from build123d import *

# Parameters (mm, degrees)
BOSS_EXTRUDE1_DEPTH      = 11
CUT_EXTRUDE1_DEPTH       = 62.923844357
CUT_EXTRUDE1_DEPTH_BACK  = 62.923844357
SKETCH2_W                = 20.5
SKETCH2_H                = 2.6
BOSS_EXTRUDE3_START      = -8.4
BOSS_EXTRUDE3_DEPTH      = 9.4
SKETCH4_R                = 17
SKETCH4_R_2              = 10
BOSS_EXTRUDE2_DEPTH      = 5.62
SKETCH5_R                = 13.5
CUT_EXTRUDE2_DEPTH       = 4
CUT_EXTRUDE3_DEPTH       = 37.67089309
CUT_EXTRUDE3_DEPTH_BACK  = 37.67089309
SKETCH6_R                = 10.5
BOSS_EXTRUDE4_START      = 1.12
SKETCH18_R               = 17
BOSS_EXTRUDE4_DEPTH      = 1.12
CHAMFER3_SIZE            = 2.75
BOSS_EXTRUDE7_START      = 1
BOSS_EXTRUDE7_DEPTH      = 1
CUT_EXTRUDE17_START      = 12
SKETCH28_W               = 22
SKETCH28_H               = 42
CUT_EXTRUDE17_DEPTH      = 11
CUT_EXTRUDE18_DEPTH      = 37.488140539
CUT_EXTRUDE18_DEPTH_BACK = 37.488140539
SKETCH29_R               = 11
SKETCH31_R               = 1.9
CUT_EXTRUDE19_DEPTH      = 7
BOSS_EXTRUDE8_DEPTH      = 3


with BuildPart() as part:
    # Sketch1 → Boss-Extrude1 (new body)
    with BuildSketch(Plane.XY):
        with BuildLine():
            ThreePointArc((15.25, 27.5), (14.664213562, 28.914213562), (13.25, 29.5))
            Line((13.25, 29.5), (-10.25, 29.5))
            ThreePointArc((-10.25, 29.5), (-11.664213562, 28.914213562), (-12.25, 27.5))
            Line((-12.25, 27.5), (-12.25, 0.346410162))
            Line((-12.25, 0.346410162), (-12.25, 0))
            Line((-12.25, 0), (-12.25, -0.346410162))
            Line((-12.25, -0.346410162), (-12.25, -27.5))
            ThreePointArc((-12.25, -27.5), (-11.664213562, -28.914213562), (-10.25, -29.5))
            Line((-10.25, -29.5), (13.25, -29.5))
            ThreePointArc((13.25, -29.5), (14.664213562, -28.914213562), (15.25, -27.5))
            Line((15.25, -27.5), (15.25, -9.120855223))
            Line((15.25, -9.120855223), (15.25, 9.120855223))
            Line((15.25, 9.120855223), (15.25, 27.5))
        make_face()
        with BuildLine():
            Line((7, 22.5), (10.25, 22.5))
            Line((10.25, 22.5), (10.25, -22.5))
            Line((10.25, -22.5), (7, -22.5))
            Line((7, -22.5), (7, -24.7))
            ThreePointArc((7, -24.7), (5, -26.7), (3, -24.7))
            Line((3, -24.7), (3, -22.5))
            Line((3, -22.5), (-3, -22.5))
            Line((-3, -22.5), (-3, -24.7))
            ThreePointArc((-3, -24.7), (-5, -26.7), (-7, -24.7))
            Line((-7, -24.7), (-7, -22.5))
            Line((-7, -22.5), (-10.25, -22.5))
            Line((-10.25, -22.5), (-10.25, 22.5))
            Line((-10.25, 22.5), (-7, 22.5))
            Line((-7, 22.5), (-7, 24.7))
            ThreePointArc((-7, 24.7), (-5, 26.7), (-3, 24.7))
            Line((-3, 24.7), (-3, 22.5))
            Line((-3, 22.5), (3, 22.5))
            Line((3, 22.5), (3, 24.7))
            ThreePointArc((3, 24.7), (5, 26.7), (7, 24.7))
            Line((7, 24.7), (7, 22.5))
        make_face(mode=Mode.SUBTRACT)
    extrude(amount=BOSS_EXTRUDE1_DEPTH)

    # Sketch2 → Cut-Extrude1 (cut, two sides: drawn at the far end of the back side and taken through both)
    with BuildSketch(Plane(origin=(0, 29.5, 0), x_dir=(1, 0, 0), z_dir=(0, 1, 0)).offset(-CUT_EXTRUDE1_DEPTH_BACK)):
        with Locations((0, -1.3)):
            Rectangle(SKETCH2_W, SKETCH2_H)
    extrude(amount=CUT_EXTRUDE1_DEPTH + CUT_EXTRUDE1_DEPTH_BACK, mode=Mode.SUBTRACT)

    # Sketch3 → Boss-Extrude3 (add)
    with BuildSketch(Plane.XY.offset(11).offset(BOSS_EXTRUDE3_START)):
        with BuildLine():
            Line((-10.25, -29.5), (13.25, -29.5))
            ThreePointArc((13.25, -29.5), (14.664213562, -28.914213562), (15.25, -27.5))
            Line((15.25, -27.5), (15.25, 27.5))
            ThreePointArc((15.25, 27.5), (14.664213562, 28.914213562), (13.25, 29.5))
            Line((13.25, 29.5), (-10.25, 29.5))
            ThreePointArc((-10.25, 29.5), (-11.664213562, 28.914213562), (-12.25, 27.5))
            Line((-12.25, 27.5), (-12.25, -27.5))
            ThreePointArc((-12.25, -27.5), (-11.664213562, -28.914213562), (-10.25, -29.5))
        make_face()
    extrude(amount=BOSS_EXTRUDE3_DEPTH)

    # Sketch4 → Boss-Extrude2 (add)
    with BuildSketch(Plane.XY.offset(17.62)):
        with Locations((0, -11.7)):
            Circle(SKETCH4_R)
        with Locations((0, -11.7)):
            Circle(SKETCH4_R_2, mode=Mode.SUBTRACT)
    extrude(amount=-BOSS_EXTRUDE2_DEPTH)

    # Sketch5 → Cut-Extrude2 (cut)
    with BuildSketch(Plane.XY.offset(17.62)):
        with Locations((0, -11.7)):
            Circle(SKETCH5_R)
    extrude(amount=-CUT_EXTRUDE2_DEPTH, mode=Mode.SUBTRACT)

    # Sketch6 → Cut-Extrude3 (cut, two sides: drawn at the far end of the back side and taken through both)
    with BuildSketch(Plane.XY.offset(13.62).offset(-CUT_EXTRUDE3_DEPTH_BACK)):
        with Locations((0, -11.7)):
            Circle(SKETCH6_R)
    extrude(amount=CUT_EXTRUDE3_DEPTH + CUT_EXTRUDE3_DEPTH_BACK, mode=Mode.SUBTRACT)

    # Sketch18 → Boss-Extrude4 (add)
    with BuildSketch(Plane.XY.offset(12).offset(BOSS_EXTRUDE4_START)):
        with Locations((0, -11.7)):
            Circle(SKETCH18_R)
    extrude(amount=-BOSS_EXTRUDE4_DEPTH)

    # Chamfer3
    # the kernel refuses this chamfer: 2.75 mm, written as the material it adds along each edge
    with BuildSketch(Plane(origin=(0, -11.7, 12), x_dir=(0.99914018616096, 0.041459478991448445, 0), z_dir=(0.041459478991448445, -0.99914018616096, 0))) as chamfer3_piece_1_section:
        Polygon((17, CHAMFER3_SIZE), (17 + CHAMFER3_SIZE, 0), (17, 0), align=None)
    chamfer3_piece_1 = revolve(axis=Axis((0, -11.7, 12), (0, 0, 1)), revolution_arc=157.576683104, mode=Mode.PRIVATE)
    chamfer3_piece_1 = split(chamfer3_piece_1, bisect_by=Plane(origin=(15.25, 6.422467161, 13.340102963), z_dir=(-1, 0, 0)), keep=Keep.TOP, mode=Mode.PRIVATE)
    chamfer3_piece_1 = split(chamfer3_piece_1, bisect_by=Plane(origin=(-12.25, 6.422467161, 13.340102963), z_dir=(1, 0, 0)), keep=Keep.TOP, mode=Mode.PRIVATE)
    add(chamfer3_piece_1)
    with BuildSketch(Plane(origin=(0, -11.7, 12), x_dir=(-0.9394106509692863, -0.3427938576542199, 0), z_dir=(-0.3427938576542199, 0.9394106509692863, 0))) as chamfer3_piece_2_section:
        Polygon((17, CHAMFER3_SIZE), (17 + CHAMFER3_SIZE, 0), (17, 0), align=None)
    chamfer3_piece_2 = revolve(axis=Axis((0, -11.7, 12), (0, 0, 1)), revolution_arc=157.576683104, mode=Mode.PRIVATE)
    chamfer3_piece_2 = split(chamfer3_piece_2, bisect_by=Plane(origin=(15.25, -27.115392877, 14.25853692), z_dir=(-1, 0, 0)), keep=Keep.TOP, mode=Mode.PRIVATE)
    chamfer3_piece_2 = split(chamfer3_piece_2, bisect_by=Plane(origin=(-12.25, -27.115392877, 14.25853692), z_dir=(1, 0, 0)), keep=Keep.TOP, mode=Mode.PRIVATE)
    chamfer3_piece_2 = split(chamfer3_piece_2, bisect_by=Plane(origin=(-8.124246578, -29.5, 14.25853692), z_dir=(0, 1, 0)), keep=Keep.TOP, mode=Mode.PRIVATE)
    add(chamfer3_piece_2)

    # Sketch19 → Boss-Extrude7 (add)
    with BuildSketch(Plane.XY.offset(12).offset(BOSS_EXTRUDE7_START)):
        with BuildLine():
            Line((-11.360440511, 29.5), (-11.360440511, 0.946754184))
            ThreePointArc((-11.360440511, 0.946754184), (2.262558078, 5.148763484), (14.294383554, -2.498337172))
            Line((14.294383554, -2.498337172), (14.294383554, 29.5))
            Line((14.294383554, 29.5), (-11.360440511, 29.5))
        make_face()
    extrude(amount=-BOSS_EXTRUDE7_DEPTH)

    # Sketch28 → Cut-Extrude17 (cut)
    with BuildSketch(Plane(origin=(0, 0, 12), x_dir=(-1, 0, 0), z_dir=(0, 0, -1)).offset(CUT_EXTRUDE17_START)):
        Rectangle(SKETCH28_W, SKETCH28_H)
    extrude(amount=-CUT_EXTRUDE17_DEPTH, mode=Mode.SUBTRACT)

    # Sketch29 → Cut-Extrude18 (cut, two sides: drawn at the far end of the back side and taken through both)
    with BuildSketch(Plane.XY.offset(13.12).offset(-CUT_EXTRUDE18_DEPTH_BACK)):
        with Locations((0, -11.7)):
            Circle(SKETCH29_R)
    extrude(amount=CUT_EXTRUDE18_DEPTH + CUT_EXTRUDE18_DEPTH_BACK, mode=Mode.SUBTRACT)

    # Sketch31 → Cut-Extrude19 (cut)
    with BuildSketch(Plane(origin=(0, 0, 2.6), x_dir=(-1, 0, 0), z_dir=(0, 0, -1))):
        with Locations((5, 24.7)):
            Circle(SKETCH31_R)
        with Locations((-5, 24.7)):
            Circle(SKETCH31_R)
        with Locations((-5, -24.7)):
            Circle(SKETCH31_R)
        with Locations((5, -24.7)):
            Circle(SKETCH31_R)
    extrude(amount=-CUT_EXTRUDE19_DEPTH, mode=Mode.SUBTRACT)

    # Sketch35 → Boss-Extrude8 (add)
    with BuildSketch(Plane(origin=(15.25, 0, 0), x_dir=(0, 0, -1), z_dir=(1, 0, 0))):
        with BuildLine():
            Line((0, -9.120855223), (0, 9.120855223))
            ThreePointArc((0, 9.120855223), (-5.9, 0), (0, -9.120855223))
        make_face()
    extrude(amount=BOSS_EXTRUDE8_DEPTH)


solid = part.part
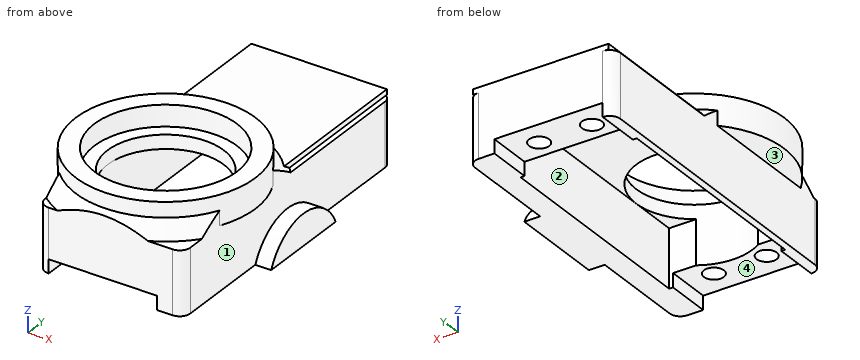
Read the model definition and answer for the solid it produces. Units are mm, in the model's axes. Face numbers are marked on the shaded views. A direction names the side the tool comes from. Coordinates: 2 decimals unless noted, no trailing zeros. Loops run counter-clockwise (first coordinate to the right, second up) from the corner with the lowest first, then second, coordinate; pieces in that order, holes last.
Q1. The part is cut by section A-A on x = 0. Write down the section's boundary in (y, z).
Q2. The part is cut by section B-B on z = 6.5. Write down the section's boundary in (x, y).
Q3. Each of these flat-tipped pins is pushed along its axis until it touches: pin 1 Ø4 at (y, z) = (-20, 5) entering from -X; pin 2 Ø0.8 at (y, z) = (-27, 1) entering from -X; pin 3 Ø1.9 at (x, y) = (5, -24) entering from -Z. Where does it stop, or does it pass through?
Q4. Consider probe 1 along X at (y, z) = (-15, 10.75); probe 2 along Y at (x, z) = (5, 8); probe 3 along X at (y, z) = (-7.5, 2). Determine where each line is inside the solid, lowest interval first.
Q5. The part is cut by section C-C on y = -14. Write down the section's boundary in (x, z).
Q6. Which of the six approach directions +Z, -Z, +X, -X, +Y, -Y give full straight-line access (tool end or side, diameter ignored) to the marked faces 1, 2, 3 and 4?
Q7. The part is cut by section D-D on y = 14. Write down the section's boundary in (x, z), and give its area (3 significant figures).
Results below:
1. outline: (-29.5, 2.6) - (-22.7, 2.6) - (-22.7, 13.62) - (-25.2, 13.62) - (-25.2, 17.62) - (-28.7, 17.62) - (-28.7, 14.75) - (-29.5, 13.95) - close; (-0.7, 11) - (21, 11) - (21, 2.6) - (29.5, 2.6) - (29.5, 13) - (7.05, 13) - (5.3, 14.75) - (5.3, 17.62) - (1.8, 17.62) - (1.8, 13.62) - (-0.7, 13.62) - close
2. outline: (-12.25, -27.5) arc R2 ccw to (-10.25, -29.5) - (13.25, -29.5) arc R2 ccw to (15.25, -27.5) - (15.25, 27.5) arc R2 ccw to (13.25, 29.5) - (-10.25, 29.5) arc R2 ccw to (-12.25, 27.5) - close; hole (-11, -21) - (-5.87, -21) arc R11 ccw to (5.87, -21) - (11, -21) - (11, 21) - (-11, 21) - close; hole circle Ø3.8 at (-5, -24.7); hole circle Ø3.8 at (-5, 24.7); hole circle Ø3.8 at (5, -24.7); hole circle Ø3.8 at (5, 24.7)
3. pin 1: stops at x = -12.25
3. pin 2: stops at x = -12.25
3. pin 3: stops at z = 9.6
4. probe 1: x = -12.25 to -11, 11 to 15.25
4. probe 2: y = -29.5 to -26.6, -22.8 to -21.5, 21 to 22.8, 26.6 to 29.5
4. probe 3: x = -12.25 to -11, 11 to 18.25
5. outline: (-16.84, 12) - (-12.25, 12) - (-12.25, 0) - (-11, 0) - (-11, 11) - (-10.76, 11) - (-10.76, 13.62) - (-13.3, 13.62) - (-13.3, 17.62) - (-16.84, 17.62) - close; (10.76, 11) - (11, 11) - (11, 0) - (15.25, 0) - (15.25, 12) - (16.84, 12) - (16.84, 17.62) - (13.3, 17.62) - (13.3, 13.62) - (10.76, 13.62) - close
6. face 1: +X
6. face 2: -Z
6. face 3: -Z, -X, +Y, -Y
6. face 4: -Z, +Y, -Y
7. outline: (-12.25, 0) - (-11, 0) - (-11, 11) - (11, 11) - (11, 0) - (15.25, 0) - (15.25, 12) - (14.29, 12) - (14.29, 13) - (-11.36, 13) - (-11.36, 12) - (-12.25, 12) - close
7. area: 114 mm2
